Verification items for the finished model (mm, model axes). Coordinates: 2 decimals unless noted, no trailing zeros. Write each loop counter-clockwise with the first axis right and the second up, starting at its lowest first coordinate (ties: lowest second). Pieces come first, ordered by that corner, then holes. Notation, with made-up numbers: (-23, 36) -> (34, 36) arc R10 ccw to (34, 42) -> close; hole circle Ø10 at (-16, -30). An arc over 180 degrees is marked (long way). Answer in a Markdown table with one row per item.
```python
from build123d import *

# Parameters (mm, degrees)
SM_BASE_FLANGE_1_DEPTH = 1
SKETCH_3_R             = 1
SKETCH_3_R_2           = 10
SKETCH_3_W             = 10
SKETCH_3_H             = 10
CUT_EXTRUDE_1_DEPTH    = 2
FILLET_1_R             = 2


# Sheet-metal steps are written as plain solids
with BuildPart() as part:
    # Sketch 1 → 基材-凸緣1 (new body)
    with BuildSketch(Plane.XY):
        Polygon((-69.55, 38.6), (69.55, 38.6), (69.55, 28.5), (51.5, -20), (-51.5, -20), (-69.55, 28.5), align=None)
    extrude(amount=-SM_BASE_FLANGE_1_DEPTH)

    # 草圖3 → 除料-伸長1 (cut)
    with BuildSketch(Plane.XY):
        with Locations((0, -15)):
            Circle(SKETCH_3_R)
        with Locations((44, -15)):
            Circle(SKETCH_3_R)
        with Locations((-44, -15)):
            Circle(SKETCH_3_R)
        with Locations((-50.81612653, -7.502401461)):
            Circle(SKETCH_3_R)
        with Locations((-61.977500026, 22.487992696)):
            Circle(SKETCH_3_R)
        with Locations((0, 33.6)):
            Circle(SKETCH_3_R)
        with Locations((-26, 33.6)):
            Circle(SKETCH_3_R)
        with Locations((-52, 33.6)):
            Circle(SKETCH_3_R)
        with Locations((26, 33.6)):
            Circle(SKETCH_3_R)
        with Locations((52, 33.6)):
            Circle(SKETCH_3_R)
        with Locations((61.977500026, 22.487992696)):
            Circle(SKETCH_3_R)
        with Locations((50.81612653, -7.502401461)):
            Circle(SKETCH_3_R)
        with Locations((-41.112999651, 18.6)):
            Circle(SKETCH_3_R_2)
        with Locations((41.112999651, 18.6)):
            Circle(SKETCH_3_R_2)
        with Locations((-64.55, 33.6)):
            Rectangle(SKETCH_3_W, SKETCH_3_H)
        with Locations((64.55, 33.6)):
            Rectangle(SKETCH_3_W, SKETCH_3_H)
    extrude(amount=-CUT_EXTRUDE_1_DEPTH, mode=Mode.SUBTRACT)

    # 圓角1
    fillet_1_edges = [part.edges().sort_by_distance(p)[0] for p in [
        (51.5, -20, -0.5),
        (-51.5, -20, -0.5),
        (59.55, 38.6, -0.5),
        (-59.55, 38.6, -0.5),
    ]]
    fillet(fillet_1_edges, radius=FILLET_1_R)


solid = part.part
```
1. Material ranges on probe 1 along Y at (x, z) = (0, -0.4); probe 2 along X at (y, z) = (19, -0.75) (3 decimals); probe 3 along X at (y, z) = (14, -0.3), recorded low to high. Write a range as from..to.
Findings below:
| item | result |
|---|---|
| probe 1 | y = -20..-16, -14..32.6, 34.6..38.6 |
| probe 2 | x = -66.014..-51.105, -31.121..31.121, 51.105..66.014 |
| probe 3 | x = -64.15..-49.99, -32.23..32.23, 49.99..64.15 |
2. Release check for a two-part mould opening along Y. For faces 1 (the face through (1, 10, 0)), 2 (the face through (-60.644, 4.571, -0.493)), 3 (the face through (33.177, 12.515, -0.493)) record: released by +Y, released by -Y, zero draft, split by the parting line, or undercut.
Findings below:
| item | result |
|---|---|
| face 1 | zero draft |
| face 2 | released by -Y |
| face 3 | undercut |
3. Sectioned sample at C-C, the plane z = -0.15. Count the separate pieces of the cut face and the enclosed holes in it, and give its area (3 significant figures).
Findings below:
| item | result |
|---|---|
| separate pieces | 1 |
| enclosed holes | 14 |
| area | 6,410 mm² |
4. Sectioned sample at A-A, the plane y = 27. Record the cut outline in (x, z).
Findings below:
| item | result |
|---|---|
| outline | (-68.99, -1) -> (-46.54, -1) -> (-46.54, 0) -> (-68.99, 0) -> close; (-35.69, -1) -> (35.69, -1) -> (35.69, 0) -> (-35.69, 0) -> close; (46.54, -1) -> (68.99, -1) -> (68.99, 0) -> (46.54, 0) -> close |
5. Sectioned sample at D-D, the plane y = 18.6. Record the cut outline in (x, z).
Findings below:
| item | result |
|---|---|
| outline | (-65.87, -1) -> (-51.11, -1) -> (-51.11, 0) -> (-65.87, 0) -> close; (-31.11, -1) -> (31.11, -1) -> (31.11, 0) -> (-31.11, 0) -> close; (51.11, -1) -> (65.87, -1) -> (65.87, 0) -> (51.11, 0) -> close |
6. Sectioned sample at B-B, the plane x = -48.5. Record the cut outline in (y, z).
Findings below:
| item | result |
|---|---|
| outline | (-20, -1) -> (11.86, -1) -> (11.86, 0) -> (-20, 0) -> close; (25.34, -1) -> (38.6, -1) -> (38.6, 0) -> (25.34, 0) -> close |
7. Go/stop test with flat-tipped pins: pin 1 (0.5 mm diameter, centred on x = -64.5, z = -0.5, fed in from +Y); pin 2 (2.5 mm diameter, centred on x = -52, y = 33.6, fed in from +Z). Record where each tip stops, or that it passes through.
Findings below:
| item | result |
|---|---|
| pin 1 | stops at y = 28.6 |
| pin 2 | stops at z = 0 |
